Part model, mm, in its own coordinate system. Round coordinates to 2 decimals unless told otherwise and drop trailing zeros. Write each loop counter-clockwise with the first axis right and the second up, starting at its lowest first coordinate (ties: lowest second). Pieces come first, ordered by that corner, then holes. Notation, with made-up numbers: M -1,20.5 L 15,20.5 A15 ccw 15,36.5 Z; hole C 2.5,17.5 d10. An arc over 180 degrees is marked long. Answer as a JSON object with one key per item and string values. Group by question number.
1. Drop flat-ended pins along their axis: pin 1 (1 mm diameter, centred on y = 12.5, z = 1, fed in from -X); pin 2 (10 mm diameter, centred on x = 27.5, y = 37, fed in from -Z); pin 3 (0.9 mm diameter, centred on x = 1.5, z = 1, fed in from -Y); pin 4 (1.5 mm diameter, centred on x = -1.5, z = 1.5, fed in from -Y). Give the stop position or say it passes through.
2. Band-saw the part on A-A, the plane y = 42.5. Write the cut outline in (x, z).
3. Band-saw the part on B-B, the plane z = 0.95. Write the cut outline in (x, y), plus the area to 3 significant figures.
4. Band-saw the part on D-D, the plane x = 139. Write the cut outline in (y, z), plus the area to 3 significant figures.
5. Band-saw the part on C-C, the plane y = 31.5. Write the cut outline in (x, z).
6. Drill centre lines: line 1 (X direction, y = 31.5, z = 1.45); line 2 (X direction, y = 59, z = 2.65); line 3 (X direction, y = 16.5, z = 0.9). Where is each one in solid material? Low to high. Write a range as from..to.
Autodesk Inventor part; units mm, degrees
ref_plane "YZ Plane" through (0, 0, 0) normal (1, 0, 0) x (0, 1, 0)
ref_plane "XZ Plane" through (0, 0, 0) normal (0, 1, 0) x (-1, 0, 0)
ref_plane "XY Plane" through (0, 0, 0) normal (0, 0, 1) x (1, 0, 0)
sketch "Sketch1" plane through (0, 0, 0) normal (0, 0, 1) x (1, 0, 0)
  line L0 (0, 0) -> (171.704, 0)
  line L1 (171.704, 0) -> (171.704, 63.5)
  line L2 (171.704, 63.5) -> (0, 63.5)
  line L3 (0, 63.5) -> (0, 0)
  arc A0 (0, 25.4) -> (25.4, 0) centre (25.4, 25.4) ccw
  arc A1 (146.304, 0) -> (171.704, 25.4) centre (146.304, 25.4) ccw
  dimension "d0" = 171.704
  dimension "d1" = 63.5
  dimension "d2" = 50.8
  dimension "d3" = 50.8
extrude "Extrusion1" add sketch "Sketch1" along normal blind 3.048 contours A0 L3 L2 L1 A1 L0
sketch "Sketch3" plane through (0, 25.4, 0) normal (-1, 0, 0) x (0, 0, 1)
  line L0 (0, 38.1) -> (0, 0)
  line L1 (3.048, -25.4) -> (3.048, 0)
  line L2 (0, 38.1) -> (3.048, 38.1)
  line L3 (3.048, 38.1) -> (3.048, 0)
  line L4 (3.048, 0) -> (0, 0)
  line L5 (0, 0) -> (0, 38.1)
  point P0 (0, -25.4)
extrude "Extrusion3" add sketch "Sketch3" along normal blind 3.048
sketch "Sketch4" plane through (171.704, 25.4, 0) normal (1, 0, 0) x (0, 0, -1)
  line L0 (-3.048, 38.1) -> (0, 38.1)
  line L1 (0, 0) -> (0, -25.4)
  line L2 (-3.048, 38.1) -> (0, 38.1)
  line L3 (0, 38.1) -> (0, 0)
  line L4 (0, 0) -> (-3.048, 0)
  line L5 (-3.048, 0) -> (-3.048, 38.1)
  point P0 (0, -25.4)
extrude "Extrusion4" add sketch "Sketch4" along normal blind 3.048
sketch "Sketch5" plane through (0, 0, 3.048) normal (0, 0, 1) x (1, 0, 0)
  line L0 (0, 0) -> (3.048, 0)
  line L1 (3.048, 0) -> (3.048, 38.1)
  line L2 (3.048, 38.1) -> (0, 38.1)
  line L3 (0, 38.1) -> (0, 0)
  line L4 (-3.048, 63.5) -> (174.752, 63.5)
  line L5 (85.852, 63.5) -> (85.852, 0)
  line L6 (25.4, 0) -> (146.304, 0)
  line L7 (171.704, 0) -> (168.656, 0)
  line L8 (168.656, 0) -> (168.656, 38.1)
  line L9 (168.656, 38.1) -> (171.704, 38.1)
  line L10 (171.704, 38.1) -> (171.704, 0)
  point P0 (1.524, 0)
  point P1 (170.18, 0)
  dimension "d17" = 38.1
  dimension "d18" = 3.048
extrude "Extrusion5" cut sketch "Sketch5" against normal through all
sketch "Sketch6" plane through (0, 0, 3.048) normal (0, 0, 1) x (1, 0, 0)
  line L0 (-3.048, 63.5) -> (174.752, 63.5)
  line L1 (22.098, 63.5) -> (149.606, 63.5)
  line L2 (149.606, 63.5) -> (149.606, 25.4)
  line L3 (149.606, 25.4) -> (22.098, 25.4)
  line L4 (22.098, 25.4) -> (22.098, 63.5)
  line L5 (3.048, 38.1) -> (3.048, 13.3357)
  line L6 (168.656, 13.3357) -> (168.656, 38.1)
  line L7 (25.4, 0) -> (146.304, 0)
  point P0 (0, 0)
  point P1 (149.606, 63.5)
  dimension "d21" = 19.05
  dimension "d22" = 19.05
  dimension "d23" = 25.4
extrude "Extrusion6" cut sketch "Sketch6" against normal through all
properties part number "Battery_container_main"
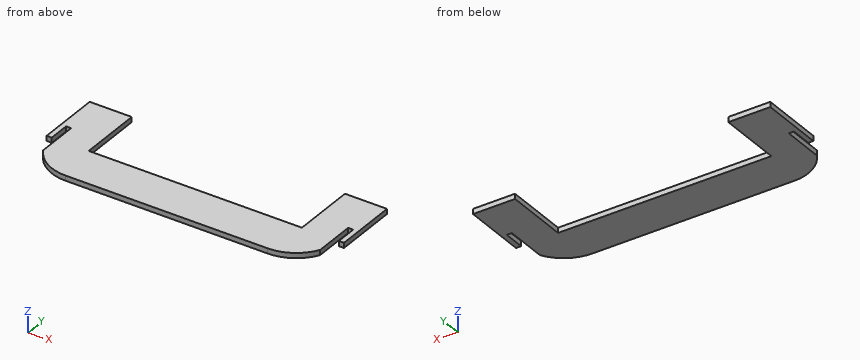
Worked answers:
{
 "1": {"pin 1": "stops at x = 3.23", "pin 2": "passes through", "pin 3": "stops at y = 38.1", "pin 4": "stops at y = 25.4"},
 "2": {"outline": "M -3.05,0 L 22.1,0 L 22.1,3.05 L -3.05,3.05 Z; M 149.61,0 L 174.75,0 L 174.75,3.05 L 149.61,3.05 Z"},
 "3": {"outline": "M -3.05,25.4 L 0,25.4 L 0,38.1 L 3.05,38.1 L 3.05,13.34 A25.4 ccw 25.4,0 L 146.3,0 A25.4 ccw 168.66,13.34 L 168.66,38.1 L 171.7,38.1 L 171.7,25.4 L 174.75,25.4 L 174.75,63.5 L 149.61,63.5 L 149.61,25.4 L 22.1,25.4 L 22.1,63.5 L -3.05,63.5 Z", "area": "5,870 mm^2"},
 "4": {"outline": "M 0,0 L 25.4,0 L 25.4,3.05 L 0,3.05 Z", "area": "77.4 mm^2"},
 "5": {"outline": "M -3.05,0 L 0,0 L 0,3.05 L -3.05,3.05 Z; M 3.05,0 L 22.1,0 L 22.1,3.05 L 3.05,3.05 Z; M 149.61,0 L 168.66,0 L 168.66,3.05 L 149.61,3.05 Z; M 171.7,0 L 174.75,0 L 174.75,3.05 L 171.7,3.05 Z"},
 "6": {"line 1": "x = -3.05..0, 3.05..22.1, 149.61..168.66, 171.7..174.75", "line 2": "x = -3.05..22.1, 149.61..174.75", "line 3": "x = 3.05..168.66"}
}
